Verification items for this drawing (mm, ordinates from the low corner). Round coordinates to 2 decimals unless told otherwise and drop trailing zeros. Loops run counter-clockwise (first coordinate to the right, second up) from the corner with the lowest first, then second, coordinate; pieces in that order, holes last. Notation, with made-up numbers: (-30.75, 55.25) -> (9.25, 55.25) arc R22 ccw to (9.25, 75.25) -> close; hole circle Ø5 at (-30.5, -1). An arc over 180 degrees is marked (long way). Use a Markdown table: item, result. Add a question column.
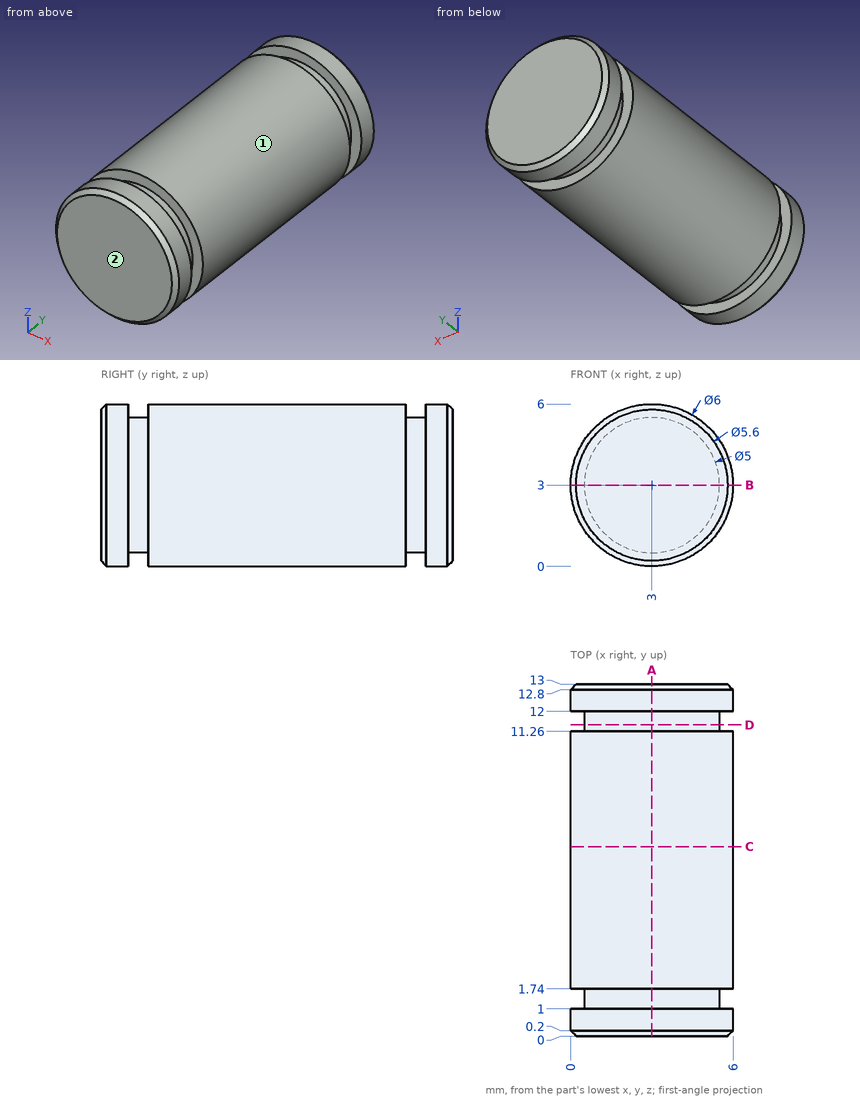
1) Sectioned sample at D-D on y = 11.5. Enter the section's corners in (x, z).
2) Sectioned sample at A-A on x = 3. Enter the section's corners in (y, z).
3) Thickness scan on line 1 (Y direction, x = 1.2, z = 5.1); line 2 (X direction, y = 9.5, z = 0.3); line 3 (X direction, y = 2.5, z = 2.75). Record the ranges inside material, lowest first.
4) Sectioned sample at B-B on z = 3. Enter the section's corners in (x, y), then the cut area to 3 significant figures.
5) Go/stop test with a flat-tipped pin: pin 1 (2 mm diameter, centred on y = 5.5, z = 5, fed in from +X). Record where the tip stops, or that it passes through.
6) Release check for a two-part mould opening along X. For the marked faces 1 and 2 record: released by +X, released by -X, zero draft, split by the parting line, or undercut.
7) Sectioned sample at C-C on y = 7. Enter the section's corners in (x, z), then the cut area to 3 significant figures.
Geometry results:
| question | item | result |
|---|---|---|
| 1 | outline | circle Ø5 at (3, 3) |
| 2 | outline | (0, 0.2) -> (0.2, 0) -> (1, 0) -> (1, 0.5) -> (1.74, 0.5) -> (1.74, 0) -> (11.26, 0) -> (11.26, 0.5) -> (12, 0.5) -> (12, 0) -> (12.8, 0) -> (13, 0.2) -> (13, 5.8) -> (12.8, 6) -> (12, 6) -> (12, 5.5) -> (11.26, 5.5) -> (11.26, 6) -> (1.74, 6) -> (1.74, 5.5) -> (1, 5.5) -> (1, 6) -> (0.2, 6) -> (0, 5.8) -> close |
| 3 | line 1 | 0 to 1, 1.74 to 11.26, 12 to 13 |
| 3 | line 2 | 1.69 to 4.31 |
| 3 | line 3 | 0.01 to 5.99 |
| 4 | outline | (0, 0.2) -> (0.2, 0) -> (5.8, 0) -> (6, 0.2) -> (6, 1) -> (5.5, 1) -> (5.5, 1.74) -> (6, 1.74) -> (6, 11.26) -> (5.5, 11.26) -> (5.5, 12) -> (6, 12) -> (6, 12.8) -> (5.8, 13) -> (0.2, 13) -> (0, 12.8) -> (0, 12) -> (0.5, 12) -> (0.5, 11.26) -> (0, 11.26) -> (0, 1.74) -> (0.5, 1.74) -> (0.5, 1) -> (0, 1) -> close |
| 4 | area | 76.4 mm^2 |
| 5 | pin 1 | x = 5.83 |
| 6 | face 1 | split by the parting line |
| 6 | face 2 | zero draft |
| 7 | outline | circle Ø6 at (3, 3) |
| 7 | area | 28.3 mm^2 |
